Input: part model. Units: mm. Frame: model coordinates. Face numbers are marked on the shaded views. Coordinates: 2 decimals unless noted, no trailing zeros. Loops run counter-clockwise (first coordinate to the right, second up) from the corner with the lowest first, then second, coordinate; pieces in that order, holes last.
(1) Section A-A, the plane y = 0. Return loops of the section in (x, z).
(2) Section B-B, the plane z = 2.25. Return loops of the section in (x, y).
(3) Contact query for flat-ended pins moving along their axis: P1, Ø2, axis at y = 2, z = 18, coming from the +X side; P2, Ø1.8, axis at x = 0, y = -0.5, coming from the -Z side; P3, Ø1, axis at y = 2.5, z = 10.5, coming from the +X side. Output: stop coordinate, or through.
(4) Line query: L1, parallel to Y at x = 0, z = 1.8; L2, parallel to Z at x = -0.5, y = 1; L3, parallel to Y at x = 1.25, z = 9.5. Output: solid intervals per line, ascending.
(5) Section D-D, the plane z = 15.25. Return loops of the section in (x, y).
(6) Mould query, pull axis Y, two halves, no side actions, for the marked faces 1, 2 and 3. Classes: released by +Y, released by -Y, zero draft, split by the parting line, or undercut.
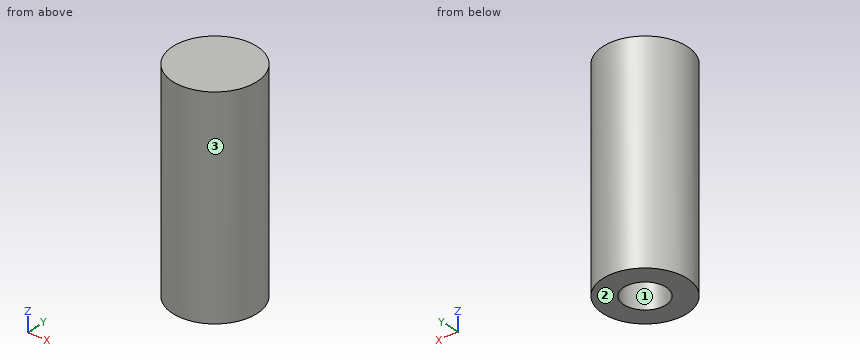
```python
from build123d import *

# Parameters (mm, degrees)
ESQUISSE1_R             = 4
BOSS_EXTRU_1_DEPTH      = 20
ESQUISSE2_R             = 1.75
ENL_V_MAT_EXTRU_1_DEPTH = 10
ESQUISSE3_R             = 2
ENL_V_MAT_EXTRU_2_DEPTH = 5


with BuildPart() as part:
    # Esquisse1 → Boss.-Extru.1 (new body)
    with BuildSketch(Plane.XY):
        Circle(ESQUISSE1_R)
    extrude(amount=BOSS_EXTRU_1_DEPTH)

    # Esquisse2 → Enlèv. mat.-Extru.1 (cut)
    with BuildSketch(Plane(origin=(0, 0, 0), x_dir=(-1, 0, 0), z_dir=(0, 0, -1))):
        Circle(ESQUISSE2_R)
    extrude(amount=-ENL_V_MAT_EXTRU_1_DEPTH, mode=Mode.SUBTRACT)

    # Esquisse3 → Enlèv. mat.-Extru.2 (cut)
    with BuildSketch(Plane(origin=(0, 0, 0), x_dir=(-1, 0, 0), z_dir=(0, 0, -1))):
        Circle(ESQUISSE3_R)
    extrude(amount=-ENL_V_MAT_EXTRU_2_DEPTH, mode=Mode.SUBTRACT)


solid = part.part
```
Report:
1. outline: (-4, 0) - (-2, 0) - (-2, 5) - (-1.75, 5) - (-1.75, 10) - (1.75, 10) - (1.75, 5) - (2, 5) - (2, 0) - (4, 0) - (4, 20) - (-4, 20) - close
2. outline: circle Ø8 at (0, 0); hole circle Ø4 at (0, 0)
3. P1: stops at x = 3.87
3. P2: stops at z = 10
3. P3: stops at x = 3.46
4. L1: y = -4 to -2, 2 to 4
4. L2: z = 10 to 20
4. L3: y = -3.8 to -1.22, 1.22 to 3.8
5. outline: circle Ø8 at (0, 0)
6. face 1: undercut
6. face 2: zero draft
6. face 3: split by the parting line
